CAD build for the part. Positions are in the model's coordinates, mm. Face numbers are marked on the shaded views. A direction names the side the tool comes from. Round coordinates to 2 decimals unless told otherwise and drop trailing zeros. Write each loop counter-clockwise with the first axis right and the second up, starting at its lowest first coordinate (ties: lowest second). Pieces come first, ordered by that corner, then holes. Notation, with made-up numbers: (50, 41) -> (55, 41) arc R24 ccw to (55, 79) -> close; hole circle Ø7 at (-29.75, 35). An arc over 180 degrees is marked (long way). Put each result on its own line as item: value. Start each with the question number.
1. 3-axis set-ups, long thin cutter, end or side, ignore diameter. For the marked faces 4, 5 and 6: which of +Z, -Z, +X, -X, +Y, -Y reach the whole face in a straight line?
2. Saw through at B-B on x = 24.5. State how many separate pieces and enclosed holes the cut face has, and give its area (3 significant figures).
3. Saw through at C-C on y = 12. List the corners of the cut face in (x, z), and give its area (3 significant figures).
4. Saw through at A-A on z = -2. List the corners of the cut face in (x, y).
5. Drill centre lines: line 1 (Y direction, x = 28, z = -9); line 2 (X direction, y = -0.75, z = -6); line 3 (Y direction, x = 38, z = 3). Where is each one in solid material? Low to high. Write a range as from..to.
6. Flat gauge pins, fed straight in: P1, Ø6, axis at x = 17.5, z = -4.5, coming from the -Y side; P2, Ø5, axis at x = 8.5, y = -59.5, coming from the +Z side; P3, Ø4.5, axis at x = 24.5, z = -6, coming from the +Y side. Where does each tip first touch, or does it go through?
7. Pull direction Y, two halves, no side cores. Call the marked faces 1, 2 and 3: pulls with the +Y half, pulls with the -Y half, needs draft (parallel to the pull), parting line crosses it, or undercut.
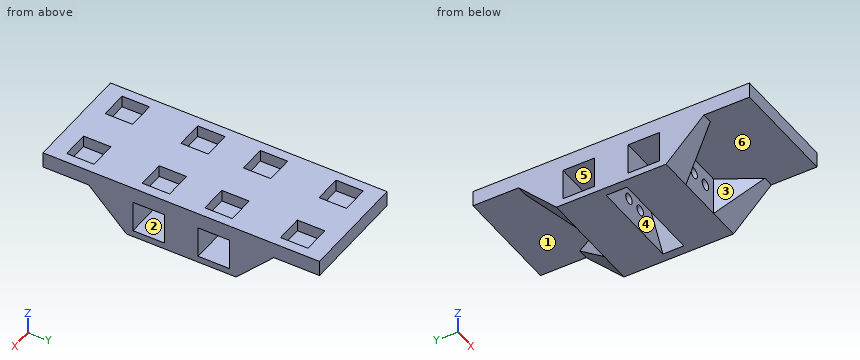
from build123d import *

# Parameters (mm, degrees)
ESQUISSE1_W                  = 42
ESQUISSE1_H                  = 106
BOSS_EXTRU_1_DEPTH           = 6
ESQUISSE2_W                  = 42
ESQUISSE2_H                  = 17
BOSS_EXTRU_3_DEPTH           = 14.5
ESQUISSE3_W                  = 12
ESQUISSE3_H                  = 12
ENL_V_MAT_EXTRU_3_DEPTH      = 87.314830707
ESQUISSE4_R                  = 2
ENL_V_MAT_EXTRU_4_DEPTH      = 42
ESQUISSE5_W                  = 10.5
ESQUISSE5_H                  = 10.5
ENL_V_MAT_EXTRU_5_DEPTH      = 4.5
SYM_TRIE3_COPY_1_SKETCH_W    = 10.5
SYM_TRIE3_COPY_1_SKETCH_H    = 10.5
SYM_TRIE3_COPY_1_DEPTH       = 4.5
SYM_TRIE4_COPY_1_SKETCH_W    = 10.5
SYM_TRIE4_COPY_1_SKETCH_H    = 10.5
SYM_TRIE4_COPY_1_DEPTH       = 4.5
SYM_TRIE5_COPY_1_SKETCH_W    = 10.5
SYM_TRIE5_COPY_1_SKETCH_H    = 10.5
SYM_TRIE5_COPY_1_DEPTH       = 4.5
SYM_TRIE5_COPY_2_SKETCH_W    = 10.5
SYM_TRIE5_COPY_2_SKETCH_H    = 10.5
SYM_TRIE5_COPY_2_DEPTH       = 4.5
SYM_TRIE5_COPY_3_SKETCH_W    = 10.5
SYM_TRIE5_COPY_3_SKETCH_H    = 10.5
SYM_TRIE5_COPY_3_DEPTH       = 4.5
BOSS_EXTRU_4_DEPTH           = 4
BOSS_EXTRU_5_REACH           = 88.315
R_P_TITION_CIRCULAIRE1_COUNT = 2
SYM_TRIE6_COPY_1_DEPTH       = 4
SYM_TRIE6_COPY_2_REACH       = 88.315
ESQUISSE8_W                  = 12
ESQUISSE8_H                  = 8
BOSS_EXTRU_6_DEPTH           = 14.5
CHANFREIN2_SIZE              = 15
CHANFREIN2_SIZE_2            = 8.660254038
SYM_TRIE7_START              = -25
SYM_TRIE7_DEPTH              = 8


# Read off the part's stored shape, not the designer's step: Symétrie7
with BuildPart() as part:
    # Esquisse1 → Boss.-Extru.1 (new body)
    with BuildSketch(Plane.XY):
        with Locations((21, -21)):
            Rectangle(ESQUISSE1_W, ESQUISSE1_H)
    extrude(amount=BOSS_EXTRU_1_DEPTH)

    # Esquisse2 → Boss.-Extru.3 (add)
    with BuildSketch(Plane(origin=(0, 0, 0), x_dir=(-1, 0, 0), z_dir=(0, 0, -1))):
        with Locations((-21, -33.5)):
            Rectangle(ESQUISSE2_W, ESQUISSE2_H)
    boss_extru_3 = extrude(amount=BOSS_EXTRU_3_DEPTH)

    # Esquisse3 → Enlèv. mat.-Extru.3 (cut, through all)
    with BuildSketch(Plane(origin=(42, 0, 0), x_dir=(0, 0, -1), z_dir=(1, 0, 0))):
        with Locations((6, -33.5)):
            Rectangle(ESQUISSE3_W, ESQUISSE3_H)
    enl_v_mat_extru_3 = extrude(amount=-ENL_V_MAT_EXTRU_3_DEPTH, mode=Mode.SUBTRACT)

    # Symétrie1: Boss.-Extru.3, Enlèv. mat.-Extru.3 across plane
    add(boss_extru_3.mirror(Plane(origin=(0, -21, 0), x_dir=(0, 0, 1), z_dir=(0, -1, 0))))
    add(enl_v_mat_extru_3.mirror(Plane(origin=(0, -21, 0), x_dir=(0, 0, 1), z_dir=(0, -1, 0))), mode=Mode.SUBTRACT)

    # Esquisse4 → Enlèv. mat.-Extru.4 (cut)
    with BuildSketch(Plane.XZ.offset(42)):
        with Locations(Location((24.5, -6, 0), (0, 0, 270))):
            Circle(ESQUISSE4_R)
        with Locations(Location((17.5, -6, 0), (0, 0, 270))):
            Circle(ESQUISSE4_R)
    extrude(amount=-ENL_V_MAT_EXTRU_4_DEPTH, mode=Mode.SUBTRACT)

    # Esquisse5 → Enlèv. mat.-Extru.5 (cut)
    with BuildSketch(Plane.XY.offset(6)):
        with Locations((9, -9)):
            Rectangle(ESQUISSE5_W, ESQUISSE5_H)
    enl_v_mat_extru_5 = extrude(amount=-ENL_V_MAT_EXTRU_5_DEPTH, mode=Mode.SUBTRACT)

    # Symétrie2: Enlèv. mat.-Extru.5 across plane
    add(enl_v_mat_extru_5.mirror(Plane(origin=(21, 0, 0), x_dir=(0, 0, 1), z_dir=(1, 0, 0))), mode=Mode.SUBTRACT)

    # Symétrie3: Enlèv. mat.-Extru.5 across plane
    add(enl_v_mat_extru_5.mirror(Plane(origin=(0, -21, 0), x_dir=(0, 0, 1), z_dir=(0, -1, 0))), mode=Mode.SUBTRACT)

    # Symétrie3 copy 1 sketch → Symétrie3 copy 1 (cut)
    with BuildSketch(Plane(origin=(42, -42, 6), x_dir=(-1, 0, 0), z_dir=(0, 0, 1))):
        with Locations((9, -9)):
            Rectangle(SYM_TRIE3_COPY_1_SKETCH_W, SYM_TRIE3_COPY_1_SKETCH_H)
    extrude(amount=-SYM_TRIE3_COPY_1_DEPTH, mode=Mode.SUBTRACT)

    # Symétrie4: Enlèv. mat.-Extru.5 across plane
    add(enl_v_mat_extru_5.mirror(Plane(origin=(0, 5.5, 0), x_dir=(0, 0, 1), z_dir=(0, -1, 0))), mode=Mode.SUBTRACT)

    # Symétrie4 copy 1 sketch → Symétrie4 copy 1 (cut)
    with BuildSketch(Plane(origin=(42, 11, 6), x_dir=(-1, 0, 0), z_dir=(0, 0, 1))):
        with Locations((9, -9)):
            Rectangle(SYM_TRIE4_COPY_1_SKETCH_W, SYM_TRIE4_COPY_1_SKETCH_H)
    extrude(amount=-SYM_TRIE4_COPY_1_DEPTH, mode=Mode.SUBTRACT)

    # Symétrie5 copy 1 sketch → Symétrie5 copy 1 (cut)
    with BuildSketch(Plane(origin=(0, -53, 6), x_dir=(1, 0, 0), z_dir=(0, 0, 1))):
        with Locations((9, -9)):
            Rectangle(SYM_TRIE5_COPY_1_SKETCH_W, SYM_TRIE5_COPY_1_SKETCH_H)
    extrude(amount=-SYM_TRIE5_COPY_1_DEPTH, mode=Mode.SUBTRACT)

    # Symétrie5 copy 2 sketch → Symétrie5 copy 2 (cut)
    with BuildSketch(Plane(origin=(42, -53, 6), x_dir=(-1, 0, 0), z_dir=(0, 0, 1))):
        with Locations((9, 9)):
            Rectangle(SYM_TRIE5_COPY_2_SKETCH_W, SYM_TRIE5_COPY_2_SKETCH_H)
    extrude(amount=-SYM_TRIE5_COPY_2_DEPTH, mode=Mode.SUBTRACT)

    # Symétrie5 copy 3 sketch → Symétrie5 copy 3 (cut)
    with BuildSketch(Plane(origin=(0, -95, 6), x_dir=(1, 0, 0), z_dir=(0, 0, 1))):
        with Locations((9, 9)):
            Rectangle(SYM_TRIE5_COPY_3_SKETCH_W, SYM_TRIE5_COPY_3_SKETCH_H)
    extrude(amount=-SYM_TRIE5_COPY_3_DEPTH, mode=Mode.SUBTRACT)

    # Esquisse6 → Boss.-Extru.4 (add)
    with BuildSketch(Plane.ZY):
        Polygon((-14.5, -42), (0, -56.5), (0, -42), align=None)
    boss_extru_4 = extrude(amount=-BOSS_EXTRU_4_DEPTH)

    # Boss.-Extru.5: up to this face of the body (flat: up to its plane)
    boss_extru_5_end = Plane(part.part.faces().sort_by_distance((2, -49.25, -7.25))[0])
    # Esquisse7 → Boss.-Extru.5 (add, up to the picked face)
    with BuildSketch(Plane(origin=(0, 0, 0), x_dir=(-1, 0, 0), z_dir=(0, 0, -1)), mode=Mode.PRIVATE) as boss_extru_5_sk1:
        Polygon((-4, -56.5), (-12.371578903, -42), (-4, -42), align=None)
    boss_extru_5_tool1 = split(extrude(boss_extru_5_sk1.sketch, amount=BOSS_EXTRU_5_REACH, mode=Mode.PRIVATE), bisect_by=boss_extru_5_end, keep=Keep.BOTH, mode=Mode.PRIVATE)
    boss_extru_5 = boss_extru_5_tool1.solids().sort_by(Axis((6.790526, -46.833333, 0), (0, 0, -1)))[0]
    add(boss_extru_5)

    # Répétition circulaire1: Boss.-Extru.4, Boss.-Extru.5 ×2 about axis
    r_p_tition_circulaire1_axis = Axis((21, -21, 0), (0, 0, 1))
    add([boss_extru_4.rotate(r_p_tition_circulaire1_axis, i * 360 / R_P_TITION_CIRCULAIRE1_COUNT) for i in range(1, R_P_TITION_CIRCULAIRE1_COUNT)])
    add([boss_extru_5.rotate(r_p_tition_circulaire1_axis, i * 360 / R_P_TITION_CIRCULAIRE1_COUNT) for i in range(1, R_P_TITION_CIRCULAIRE1_COUNT)])

    # Symétrie6: Boss.-Extru.4, Boss.-Extru.5 across plane
    add(boss_extru_4.mirror(Plane(origin=(21, 0, 0), x_dir=(0, 0, 1), z_dir=(1, 0, 0))))
    add(boss_extru_5.mirror(Plane(origin=(21, 0, 0), x_dir=(0, 0, 1), z_dir=(1, 0, 0))))

    # Symétrie6 copy 1 sketch → Symétrie6 copy 1 (add)
    with BuildSketch(Plane(origin=(0, -42, 0), x_dir=(0, 0, 1), z_dir=(-1, 0, 0))):
        Polygon((-14.5, 42), (0, 56.5), (0, 42), align=None)
    extrude(amount=-SYM_TRIE6_COPY_1_DEPTH)

    # Symétrie6 copy 2: up to this face of the body (flat: up to its plane)
    sym_trie6_copy_2_end = Plane(part.part.faces().sort_by_distance((2, 7.25, -7.25))[0])
    # Symétrie6 copy 2 sketch → Symétrie6 copy 2 (add, up to the picked face)
    with BuildSketch(Plane(origin=(0, -42, 0), x_dir=(-1, 0, 0), z_dir=(0, 0, -1)), mode=Mode.PRIVATE) as sym_trie6_copy_2_sk1:
        Polygon((-4, 56.5), (-12.371578903, 42), (-4, 42), align=None)
    sym_trie6_copy_2_tool1 = split(extrude(sym_trie6_copy_2_sk1.sketch, amount=SYM_TRIE6_COPY_2_REACH, mode=Mode.PRIVATE), bisect_by=sym_trie6_copy_2_end, keep=Keep.BOTH, mode=Mode.PRIVATE)
    add(sym_trie6_copy_2_tool1.solids().sort_by(Axis((6.790526, 4.833333, 0), (0, 0, -1)))[0])

    # Esquisse8 → Boss.-Extru.6 (add)
    with BuildSketch(Plane(origin=(0, 0, 0), x_dir=(-1, 0, 0), z_dir=(0, 0, -1))):
        with Locations((-6, -21)):
            Rectangle(ESQUISSE8_W, ESQUISSE8_H)
    extrude(amount=BOSS_EXTRU_6_DEPTH)

    # Chanfrein2
    # the kernel refuses this chamfer: 15, 8.660254038 mm, written as the material it adds along each edge
    # the kernel refuses this chamfer: 15, 8.660254038 mm, written as the material it takes off along each edge
    with BuildSketch(Plane(origin=(12, -17, -14.5), x_dir=(0.01932676561270075, 0, 0.9998132206222079), z_dir=(0, -1, 0))) as chanfrein2_2_piece_1_section:
        Polygon((CHANFREIN2_SIZE * 0.999813220622, CHANFREIN2_SIZE * 0.0193267656127), (-CHANFREIN2_SIZE_2 * 0.0193267656124, CHANFREIN2_SIZE_2 * 0.999813220604), (0, 0), align=None)
    chanfrein2_2_piece_1 = extrude(amount=8, mode=Mode.PRIVATE)
    chanfrein2_2_piece_1 = split(chanfrein2_2_piece_1, bisect_by=Plane(origin=(9.590672915, -21, 0), z_dir=(0, 0, -1)), keep=Keep.TOP, mode=Mode.PRIVATE)
    add(chanfrein2_2_piece_1, mode=Mode.SUBTRACT)

    # Symétrie7 outline → Symétrie7 (add)
    with BuildSketch(Plane(origin=(0, 0, 0), x_dir=(1, 0, 0), z_dir=(0, 1, 0)).offset(SYM_TRIE7_START)):
        Polygon((42, 0), (42, 14.5), (38.660254038, 14.5), (30.288675135, 0), align=None)
    extrude(amount=SYM_TRIE7_DEPTH)


solid = part.part
Return value:
1. face 4: -Z
1. face 5: +X, -X
1. face 6: -Z, -Y
2. separate pieces: 3
2. enclosed holes: 0
2. area: 801 mm^2
3. outline: (0, -2.5) -> (5.44, -2.5) -> (5.44, 0) -> (36.56, 0) -> (36.56, -2.5) -> (42, -2.5) -> (42, 6) -> (0, 6) -> close
3. area: 279 mm^2
4. outline: (0, -54.5) -> (5.15, -54.5) -> (12.37, -42) -> (29.63, -42) -> (36.85, -54.5) -> (42, -54.5) -> (42, -39.5) -> (0, -39.5) -> close; (0, -27.5) -> (42, -27.5) -> (42, -14.5) -> (0, -14.5) -> close; (0, -2.5) -> (42, -2.5) -> (42, 12.5) -> (36.85, 12.5) -> (29.63, 0) -> (12.37, 0) -> (5.15, 12.5) -> (0, 12.5) -> close; hole (10.56, -25) -> (31.44, -25) -> (31.44, -17) -> (10.56, -17) -> close
5. line 1: y = -42..-39.5, -27.5..-25, -17..-14.5, -2.5..0
5. line 2: x = 0..15.5, 19.5..22.5, 26.5..42
5. line 3: y = -74..-67.25, -56.75..-38.25, -27.75..-14.25, -3.75..14.75, 25.25..32
6. P1: stops at y = -42
6. P2: stops at z = 1.5
6. P3: stops at y = 0
7. face 1: needs draft
7. face 2: undercut
7. face 3: pulls with the -Y half
